Verification items for the finished model (mm, model axes). A direction names the side the tool comes from. Round coordinates to 2 decimals unless told otherwise and drop trailing zeros. Write each loop counter-clockwise with the first axis right and the second up, starting at its lowest first coordinate (ties: lowest second). Pieces come first, ordered by that corner, then holes.
from build123d import *

# Parameters (mm, degrees)
F0_R     = 10.3251
F1_DEPTH = 76.2
F3_DEPTH = 68.2625
F4_R     = 9.92251
F5_DEPTH = 88.901
F6_R     = 12.7
F7_R     = 4.7625


with BuildPart() as f1:
    # F0 (on Top) → F1 (new body)
    with BuildSketch(Plane.XY):
        with BuildLine():
            Line((0, 88.9), (0, 0))
            Line((0, 0), (57.15, 0))
            Line((57.15, 0), (57.15, 15.875))
            ThreePointArc((57.15, 15.875), (59.009872, 20.365128), (63.5, 22.225))
            Line((63.5, 22.225), (111.125, 22.225))
            ThreePointArc((111.125, 22.225), (133.35, 44.45), (111.125, 66.675))
            Line((111.125, 66.675), (63.5, 66.675))
            ThreePointArc((63.5, 66.675), (59.009872, 68.534872), (57.15, 73.025))
            Line((57.15, 73.025), (57.15, 88.9))
            Line((57.15, 88.9), (0, 88.9))
        make_face()
        with Locations((73.025, 44.45)):
            Circle(F0_R, mode=Mode.SUBTRACT)
        with Locations((111.125, 44.45)):
            Circle(F0_R, mode=Mode.SUBTRACT)
    extrude(amount=F1_DEPTH)

    # F2 (on face) → F3 (cut)
    with BuildSketch(Plane.XY.offset(76.2)):
        with BuildLine():
            ThreePointArc((57.15, 15.875), (59.009872, 20.365128), (63.5, 22.225))
            Line((63.5, 22.225), (111.125, 22.225))
            ThreePointArc((111.125, 22.225), (133.35, 44.45), (111.125, 66.675))
            Line((111.125, 66.675), (63.5, 66.675))
            ThreePointArc((63.5, 66.675), (59.009872, 68.534872), (57.15, 73.025))
            Line((57.15, 73.025), (57.15, 80.9625))
            Line((57.15, 80.9625), (0, 80.9625))
            Line((0, 80.9625), (0, 7.9502))
            Line((0, 7.9502), (57.15, 7.9502))
            Line((57.15, 7.9502), (57.15, 15.875))
        make_face()
    extrude(amount=-F3_DEPTH, mode=Mode.SUBTRACT)

    # F4 (on face) → F5 (cut, through all)
    with BuildSketch(Plane.XZ):
        with Locations((28.575, 44.45)):
            Circle(F4_R)
        with BuildLine():
            Line((0, 76.2), (0, 44.45))
            ThreePointArc((0, 44.45), (28.575, 73.025), (57.15, 44.45))
            Line((57.15, 44.45), (57.15, 76.2))
            Line((57.15, 76.2), (0, 76.2))
        make_face()
    extrude(amount=-F5_DEPTH, mode=Mode.SUBTRACT)

    # F6
    f6_edges = [f1.edges().sort_by_distance(p)[0] for p in [
        (28.575, 0, 0),
        (28.575, 88.9, 0),
    ]]
    fillet(f6_edges, radius=F6_R)

    # F7
    f7_edges = [f1.edges().sort_by_distance(p)[0] for p in [
        (28.575, 7.9502, 7.9375),
        (28.575, 80.9625, 7.9375),
    ]]
    fillet(f7_edges, radius=F7_R)


solid = f1.part
Q1. Depth check by flat-ended pin: P1, Ø3, axis at y = 9.5, z = 37, coming from the -X side; P2, Ø12, axis at y = 52, z = 12.5, coming from the +X side; P3, Ø5, axis at y = 9, z = 32, coming from the +X side; P4, Ø2.5, axis at x = 93.5, z = 4, coming from the -Y side (3 decimals). Enter the tip coordinate at first touch or a pass-through.
Recorded:
P1: passes through
P2: stops at x = 133.05
P3: stops at x = 57.15
P4: stops at y = 22.225
Q2. Sectioned sample at C-C (x = 65.5). Enter the section's corners in (y, z) (1 decimal).
Recorded:
outline: (22.2, 0) - (37.4, 0) - (37.4, 7.9) - (22.2, 7.9) - close; (51.5, 0) - (66.7, 0) - (66.7, 7.9) - (51.5, 7.9) - close
Q3. Material ranges on line 1 along X through (y, z) = (44.45, 5.25); line 2 along Z through (x, y) = (23, 55); line 3 along Y through (x, z) = (43.5, 42.5), recorded low to high.
Recorded:
line 1: x = 0 to 62.7, 83.35 to 100.8, 121.45 to 133.35
line 2: z = 0 to 7.94
line 3: y = 0 to 7.95, 80.96 to 88.9
Q4. Release check for a two-part mould opening along X. For faces 6 (the flat face through (87, 22.225, 4)), 7 (the cylindrical face through (64.83, 38.17, 3.91)), 8 (the cylindrical face through (27.95, 84.88, 73.02)), 9 (the cylindrical face through (133.345, 43.961, 3.913)) record: released by +X, released by -X, zero draft, split by the parting line, or undercut.
Recorded:
face 6: zero draft
face 7: undercut
face 8: split by the parting line
face 9: released by +X
Q5. Sectioned sample at D-D (z = 37). Enter the section's corners in (x, y).
Recorded:
outline: (0, 0) - (22.02, 0) - (22.02, 7.95) - (0, 7.95) - close; (0, 80.96) - (22.02, 80.96) - (22.02, 88.9) - (0, 88.9) - close; (35.13, 0) - (57.15, 0) - (57.15, 7.95) - (35.13, 7.95) - close; (35.13, 80.96) - (57.15, 80.96) - (57.15, 88.9) - (35.13, 88.9) - close
Q6. Tool access check on faces 1 (the flat face through (35.3, 80.962, 36.6)), 2 (the flat face through (57.15, 6, 22)), 3 (the flat face through (51, 45, 0)), 4 (the cylindrical face through (27.95, 3.92, 73.02)), 5 (the flat face through (57.15, 83, 22)). Record the directions out of +Z, -Z, +X, -X, +Y, -Y that give a thin tool (end or side, any length) a straight path to the whole face; none if there is none.
Recorded:
face 1: +Z, +X, -X
face 2: +Z, -Z, +X, -Y
face 3: -Z, +X, -X, +Y, -Y
face 4: +Z, +Y, -Y
face 5: +Z, -Z, +X, +Y
Q7. Sectioned sample at A-A (z = 25). Enter the section's corners in (x, y), plus the area to 3 significant figures.
Recorded:
outline: (0, 0) - (57.15, 0) - (57.15, 7.95) - (0, 7.95) - close; (0, 80.96) - (57.15, 80.96) - (57.15, 88.9) - (0, 88.9) - close
area: 908 mm2
Q8. Sectioned sample at B-B (y = 44.45). Enter the section's corners in (x, z), plus the area to 3 significant figures.
Recorded:
outline: (0, 0) - (62.7, 0) - (62.7, 7.94) - (0, 7.94) - close; (83.35, 0) - (100.8, 0) - (100.8, 7.94) - (83.35, 7.94) - close; (121.45, 0) - (133.35, 0) - (133.35, 7.94) - (121.45, 7.94) - close
area: 731 mm2
